Here's how the part is built. I have some questions about the finished solid (model axes, mm). A direction names the side the tool comes from. Coordinates: 2 decimals unless noted, no trailing zeros. Write each loop counter-clockwise with the first axis right and the second up, starting at its lowest first coordinate (ties: lowest second). Pieces come first, ordered by that corner, then holes. Notation, with made-up numbers: (50, -20.75) -> (81, -20.75) arc R20 cw to (81, -6.75) -> close; hole circle Ø4 at (-19.75, 4). An arc over 180 degrees is marked (long way). Use a Markdown table: item, result. Add a question column.
Item 1: Imagine slicing it at D-D, the plane x = 8.5. Write out the boundary of the cut face in (y, z), and give its area (3 significant figures).
Item 2: Imagine slicing it at A-A, the plane z = 20. Write out the boundary of the cut face in (x, y), and give its area (3 significant figures).
Item 3: Will these pins go through, and if not, where does the flat tip stop? pin 1 Ø1.5 at (y, z) = (-8.5, 2) entering from -X; pin 2 Ø4 at (x, z) = (3.5, 16) entering from -Y; pin 3 Ø3 at (x, z) = (22.5, 13.5) entering from +Y; pin 4 Ø2.5 at (y, z) = (-15, 3.5) entering from +X.
Item 4: Imagine slicing it at C-C, the plane y = 0. Write out the boundary of the cut face in (x, z).
Item 5: If we mould it in two halves opening along Y, with no side actions, what happens to faces 6 (the flat face through (25.294, -14.643, 24.65)), 7 (the flat face through (3, 0, 5)), 8 (the flat face through (3.837, 26.807, 24.65))? For each: pulls with the +Y half, pulls with the -Y half, needs draft (parallel to the pull), parting line crosses it, or undercut.
Item 6: On a 3-axis mill with a long thin cutter (end or side, diameter ignored), from which of +Z, -Z, +X, -X, +Y, -Y can I reach the whole of each face in a straight line? I mean faces 1 (the flat face through (-25.173, 10.147, 24.65)), 2 (the flat face through (0, 7, 0)), 3 (the flat face through (21, -16.727, 25)), 4 (the flat face through (-21, 16.727, 25)), 5 (the cylindrical face through (3, 4, 2)). Say none if no direction works.
Item 7: If I drill on line 1 along Y through (x, z) = (0.5, 6.5); line 2 along Y through (x, z) = (0, 2.9); line 3 along X through (y, z) = (-15.5, 4), over which ranges is the centre line in solid material (lowest first)? Write a range as from..to.
Item 8: Imagine slicing it at B-B, the plane x = 0. Write out the boundary of the cut face in (y, z).
```python
from build123d import *
from build123d.topology import SkipClean

# Parameters (mm, degrees)
SKETCH2_R           = 2.5
BOSS_EXTRUDE2_DEPTH = 5
SKETCH3_R           = 20
BOSS_EXTRUDE3_DEPTH = 45


with BuildPart() as part:
    # Sketch2 → Boss-Extrude2 (new body)
    with BuildSketch(Plane.XY):
        with BuildLine():
            ThreePointArc((-5.195852071, 24.45410234), (-12.5, 21.650635095), (-18.579947817, 16.726791058))
            Line((-18.579947817, 16.726791058), (-24.09097405, 16.726791058))
            Line((-24.09097405, 16.726791058), (-26.531313005, 12.5))
            Line((-26.531313005, 12.5), (-23.775799889, 7.727311282))
            ThreePointArc((-23.775799889, 7.727311282), (-25, 0), (-23.775799889, -7.727311282))
            Line((-23.775799889, -7.727311282), (-26.531313005, -12.5))
            Line((-26.531313005, -12.5), (-24.09097405, -16.726791058))
            Line((-24.09097405, -16.726791058), (-18.579947817, -16.726791058))
            ThreePointArc((-18.579947817, -16.726791058), (-12.5, -21.650635095), (-5.195852071, -24.45410234))
            Line((-5.195852071, -24.45410234), (-2.440338955, -29.226791058))
            Line((-2.440338955, -29.226791058), (2.440338955, -29.226791058))
            Line((2.440338955, -29.226791058), (5.195852071, -24.45410234))
            ThreePointArc((5.195852071, -24.45410234), (12.5, -21.650635095), (18.579947817, -16.726791058))
            Line((18.579947817, -16.726791058), (24.09097405, -16.726791058))
            Line((24.09097405, -16.726791058), (26.531313005, -12.5))
            Line((26.531313005, -12.5), (23.775799889, -7.727311282))
            ThreePointArc((23.775799889, -7.727311282), (25, 0), (23.775799889, 7.727311282))
            Line((23.775799889, 7.727311282), (26.531313005, 12.5))
            Line((26.531313005, 12.5), (24.09097405, 16.726791058))
            Line((24.09097405, 16.726791058), (18.579947817, 16.726791058))
            ThreePointArc((18.579947817, 16.726791058), (12.5, 21.650635095), (5.195852071, 24.45410234))
            Line((5.195852071, 24.45410234), (2.440338955, 29.226791058))
            Line((2.440338955, 29.226791058), (-2.440338955, 29.226791058))
            Line((-2.440338955, 29.226791058), (-5.195852071, 24.45410234))
        make_face()
        with BuildLine():
            Line((-16.521725449, -11.270873443), (-3.38067791, -3.683886109))
            ThreePointArc((-3.38067791, -3.683886109), (-2.5, -4.330127019), (-1.5, -4.769696007))
            Line((-1.5, -4.769696007), (-1.5, -19.943670675))
            ThreePointArc((-1.5, -19.943670675), (-10, -17.320508076), (-16.521725449, -11.270873443))
        make_face(mode=Mode.SUBTRACT)
        with BuildLine():
            Line((-18.021725449, 8.672797232), (-4.88067791, 1.085809898))
            ThreePointArc((-4.88067791, 1.085809898), (-5, 0), (-4.88067791, -1.085809898))
            Line((-4.88067791, -1.085809898), (-18.021725449, -8.672797232))
            ThreePointArc((-18.021725449, -8.672797232), (-20, 0), (-18.021725449, 8.672797232))
        make_face(mode=Mode.SUBTRACT)
        with BuildLine():
            Line((1.5, -19.943670675), (1.5, -4.769696007))
            ThreePointArc((1.5, -4.769696007), (2.5, -4.330127019), (3.38067791, -3.683886109))
            Line((3.38067791, -3.683886109), (16.521725449, -11.270873443))
            ThreePointArc((16.521725449, -11.270873443), (10, -17.320508076), (1.5, -19.943670675))
        make_face(mode=Mode.SUBTRACT)
        with BuildLine():
            Line((-1.5, 19.943670675), (-1.5, 4.769696007))
            ThreePointArc((-1.5, 4.769696007), (-2.5, 4.330127019), (-3.38067791, 3.683886109))
            Line((-3.38067791, 3.683886109), (-16.521725449, 11.270873443))
            ThreePointArc((-16.521725449, 11.270873443), (-10, 17.320508076), (-1.5, 19.943670675))
        make_face(mode=Mode.SUBTRACT)
        Circle(SKETCH2_R, mode=Mode.SUBTRACT)
        with BuildLine():
            Line((18.021725449, -8.672797232), (4.88067791, -1.085809898))
            ThreePointArc((4.88067791, -1.085809898), (5, 0), (4.88067791, 1.085809898))
            Line((4.88067791, 1.085809898), (18.021725449, 8.672797232))
            ThreePointArc((18.021725449, 8.672797232), (20, 0), (18.021725449, -8.672797232))
        make_face(mode=Mode.SUBTRACT)
        with BuildLine():
            Line((16.521725449, 11.270873443), (3.38067791, 3.683886109))
            ThreePointArc((3.38067791, 3.683886109), (2.5, 4.330127019), (1.5, 4.769696007))
            Line((1.5, 4.769696007), (1.5, 19.943670675))
            ThreePointArc((1.5, 19.943670675), (10, 17.320508076), (16.521725449, 11.270873443))
        make_face(mode=Mode.SUBTRACT)
    extrude(amount=BOSS_EXTRUDE2_DEPTH)

    # Sketch3 → Boss-Extrude3 (add)
    with SkipClean():  # the faces are left unmerged after this step: merging them gives an invalid solid
        with BuildSketch(Plane.XY.offset(5)):
            with BuildLine():
                Line((-2.440338955, 29.226791058), (-5.195852071, 24.45410234))
                ThreePointArc((-5.195852071, 24.45410234), (-12.5, 21.650635095), (-18.579947817, 16.726791058))
                Line((-18.579947817, 16.726791058), (-24.09097405, 16.726791058))
                Line((-24.09097405, 16.726791058), (-26.531313005, 12.5))
                Line((-26.531313005, 12.5), (-23.775799889, 7.727311282))
                ThreePointArc((-23.775799889, 7.727311282), (-25, 0), (-23.775799889, -7.727311282))
                Line((-23.775799889, -7.727311282), (-26.531313005, -12.5))
                Line((-26.531313005, -12.5), (-24.09097405, -16.726791058))
                Line((-24.09097405, -16.726791058), (-18.579947817, -16.726791058))
                ThreePointArc((-18.579947817, -16.726791058), (-12.5, -21.650635095), (-5.195852071, -24.45410234))
                Line((-5.195852071, -24.45410234), (-2.440338955, -29.226791058))
                Line((-2.440338955, -29.226791058), (2.440338955, -29.226791058))
                Line((2.440338955, -29.226791058), (5.195852071, -24.45410234))
                ThreePointArc((5.195852071, -24.45410234), (12.5, -21.650635095), (18.579947817, -16.726791058))
                Line((18.579947817, -16.726791058), (24.09097405, -16.726791058))
                Line((24.09097405, -16.726791058), (26.531313005, -12.5))
                Line((26.531313005, -12.5), (23.775799889, -7.727311282))
                ThreePointArc((23.775799889, -7.727311282), (25, 0), (23.775799889, 7.727311282))
                Line((23.775799889, 7.727311282), (26.531313005, 12.5))
                Line((26.531313005, 12.5), (24.09097405, 16.726791058))
                Line((24.09097405, 16.726791058), (18.579947817, 16.726791058))
                ThreePointArc((18.579947817, 16.726791058), (12.5, 21.650635095), (5.195852071, 24.45410234))
                Line((5.195852071, 24.45410234), (2.440338955, 29.226791058))
                Line((2.440338955, 29.226791058), (-2.440338955, 29.226791058))
            make_face()
            with Locations(Location((0, 0, 0), (0, 0, 154.301222305))):
                Circle(SKETCH3_R, mode=Mode.SUBTRACT)
        extrude(amount=BOSS_EXTRUDE3_DEPTH)


solid = part.part
```
Ans:
| question | item | result |
|---|---|---|
| 1 | outline | (-23.51, 0) -> (-18.1, 0) -> (-18.1, 50) -> (-23.51, 50) -> close; (-6.64, 0) -> (-3.18, 0) -> (-3.18, 5) -> (-6.64, 5) -> close; (3.18, 0) -> (6.64, 0) -> (6.64, 5) -> (3.18, 5) -> close; (18.1, 0) -> (23.51, 0) -> (23.51, 50) -> (18.1, 50) -> close |
| 1 | area | 575 mm^2 |
| 2 | outline | (-26.53, -12.5) -> (-24.09, -16.73) -> (-18.58, -16.73) arc R25 ccw to (-5.2, -24.45) -> (-2.44, -29.23) -> (2.44, -29.23) -> (5.2, -24.45) arc R25 ccw to (18.58, -16.73) -> (24.09, -16.73) -> (26.53, -12.5) -> (23.78, -7.73) arc R25 ccw to (23.78, 7.73) -> (26.53, 12.5) -> (24.09, 16.73) -> (18.58, 16.73) arc R25 ccw to (5.2, 24.45) -> (2.44, 29.23) -> (-2.44, 29.23) -> (-5.2, 24.45) arc R25 ccw to (-18.58, 16.73) -> (-24.09, 16.73) -> (-26.53, 12.5) -> (-23.78, 7.73) arc R25 ccw to (-23.78, -7.73) -> close; hole circle Ø40 at (0, 0) |
| 2 | area | 903 mm^2 |
| 3 | pin 1 | stops at x = -24.65 |
| 3 | pin 2 | stops at y = -29.23 |
| 3 | pin 3 | stops at y = 16.73 |
| 3 | pin 4 | stops at x = 25.81 |
| 4 | outline | (-25, 0) -> (-20, 0) -> (-20, 50) -> (-25, 50) -> close; (-5, 0) -> (-2.5, 0) -> (-2.5, 5) -> (-5, 5) -> close; (2.5, 0) -> (5, 0) -> (5, 5) -> (2.5, 5) -> close; (20, 0) -> (25, 0) -> (25, 50) -> (20, 50) -> close |
| 5 | face 6 | pulls with the -Y half |
| 5 | face 7 | undercut |
| 5 | face 8 | pulls with the +Y half |
| 6 | face 1 | +Z, -Z, -X |
| 6 | face 2 | -Z, +X, -X, +Y, -Y |
| 6 | face 3 | +Z, -Z, +X, -Y |
| 6 | face 4 | +Z, -Z, -X, +Y |
| 6 | face 5 | +Z, -Z |
| 7 | line 1 | y = -29.23..-19.99, 19.99..29.23 |
| 7 | line 2 | y = -29.23..-2.5, 2.5..29.23 |
| 7 | line 3 | x = -24.8..-12.64, -1.5..1.5, 12.64..24.8 |
| 8 | outline | (-29.23, 0) -> (-2.5, 0) -> (-2.5, 5) -> (-20, 5) -> (-20, 50) -> (-29.23, 50) -> close; (2.5, 0) -> (29.23, 0) -> (29.23, 50) -> (20, 50) -> (20, 5) -> (2.5, 5) -> close |
